Part print with two shaded views. Sizes in mm from the minimum x, y, z corner. Coordinates: 2 decimals unless noted, no trailing zeros. Write each loop counter-clockwise with the first axis right and the second up, starting at its lowest first coordinate (ties: lowest second). Pieces come first, ordered by that corner, then holes. Notation, with made-up numbers: (10, 60) - (60, 60) arc R16 ccw to (60, 71) - close; hole circle Ø8 at (-39.75, 64.25). An arc over 180 degrees is marked (long way). One line per question, with ' | ' between items. Start each with the question number.
1. Band-saw the part on D-D, the plane x = 18.5. Write the cut outline in (y, z).
2. Flat gauge pins, fed straight in: P1, Ø3, axis at x = 20, y = 32.5, coming from the -Z side; P2, Ø5, axis at x = 21, y = 34, coming from the -Z side. Where does each tip first touch, or does it go through?
3. Band-saw the part on C-C, the plane z = 0.65. Write the cut outline in (x, y), then the cut area to 3 significant figures.
4. Band-saw the part on B-B, the plane x = 5. Write the cut outline in (y, z).
5. Probe line 1 (X direction, y = 6, z = 1.65); line 2 (X direction, y = 34, z = 0.6); line 3 (Y direction, x = 5, z = 1.65). List the from-to ranges inside material, lowest first.
6. Band-saw the part on A-A, the plane y = 34. Write the cut outline in (x, z), then the cut area to 3 significant figures.
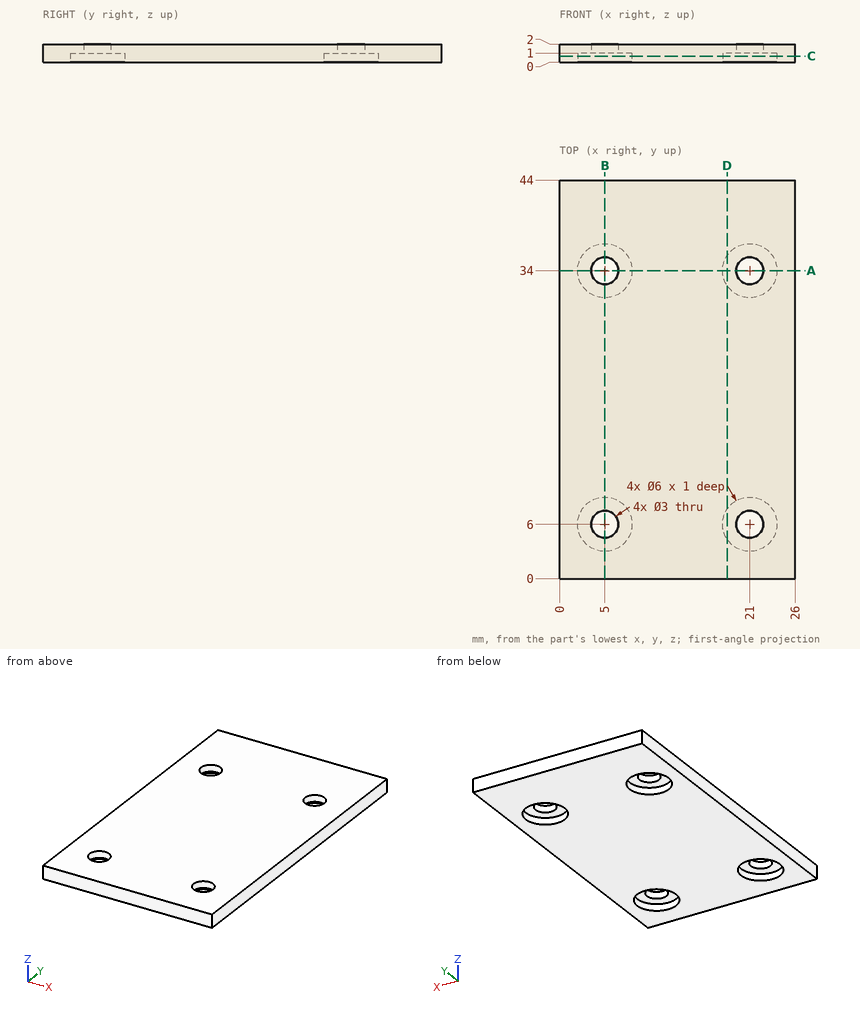
Filled in:
1) outline: (0, 0) - (4.34, 0) - (4.34, 1) - (7.66, 1) - (7.66, 0) - (32.34, 0) - (32.34, 1) - (35.66, 1) - (35.66, 0) - (44, 0) - (44, 2) - (0, 2) - close
2) P1: stops at z = 0 | P2: stops at z = 1
3) outline: (0, 0) - (26, 0) - (26, 44) - (0, 44) - close; hole circle Ø6 at (5, 6); hole circle Ø6 at (5, 34); hole circle Ø6 at (21, 6); hole circle Ø6 at (21, 34) | area: 1,030 mm²
4) outline: (0, 0) - (3, 0) - (3, 1) - (4.5, 1) - (4.5, 2) - (0, 2) - close; (7.5, 1) - (9, 1) - (9, 0) - (31, 0) - (31, 1) - (32.5, 1) - (32.5, 2) - (7.5, 2) - close; (35.5, 1) - (37, 1) - (37, 0) - (44, 0) - (44, 2) - (35.5, 2) - close
5) line 1: x = 0 to 3.5, 6.5 to 19.5, 22.5 to 26 | line 2: x = 0 to 2, 8 to 18, 24 to 26 | line 3: y = 0 to 4.5, 7.5 to 32.5, 35.5 to 44
6) outline: (0, 0) - (2, 0) - (2, 1) - (3.5, 1) - (3.5, 2) - (0, 2) - close; (6.5, 1) - (8, 1) - (8, 0) - (18, 0) - (18, 1) - (19.5, 1) - (19.5, 2) - (6.5, 2) - close; (22.5, 1) - (24, 1) - (24, 0) - (26, 0) - (26, 2) - (22.5, 2) - close | area: 34.0 mm²
